Read the model definition and answer for the solid it produces. Units are mm, in the model's axes. Face numbers are marked on the shaded views. A direction names the side the tool comes from. Coordinates: 2 decimals unless noted, no trailing zeros. Write each loop counter-clockwise with the first axis right and the second up, starting at its lowest first coordinate (ties: lowest second). Pieces come first, ordered by that corner, then holes. Notation, with made-up numbers: (-11.75, -4) -> (-0.75, -4) arc R31 cw to (-0.75, 35) -> close; hole circle Ø2 at (14.25, 6.5). An arc over 180 degrees is marked (long way). One line per item, written item: value. Start each with the question number.
1. Consider line 1 along Y through (x, z) = (120, 7.5); line 2 along X through (y, z) = (460, 8); line 3 along Y through (x, z) = (304.5, -42). Determine where each line is inside the solid, lowest interval first.
2. Find section A-A, the plane x = 120. Write down the section's boundary in (y, z).
3. Find section D-D, the plane x = 200. Write down the section's boundary in (y, z), and give its area (3 significant figures).
4. Find section C-C, the plane y = 460. Write down the section's boundary in (x, z), and give its area (3 significant figures).
5. For the marked faces 1, 2 and 3, determine the directions among +Z, -Z, +X, -X, +Y, -Y from which every point of the face is accessible in a straight line to the end or side of a thin tool.
6. Find section B-B, the plane z = -41. Write down the section's boundary in (x, y).
7. Given P1, Ø15, axis at x = 282.5, z = -16, coming from the -Y side; P2, Ø15, axis at x = 296, z = -35.5, coming from the +Y side; P3, Ø8, axis at x = 312.5, y = 414.5, coming from the -Z side; P4, Ø10, axis at x = 148.5, z = -3, coming from the +Y side, each flat-ended and moving along its own axis, determine where each tip first touches the part or whether it passes through.
Autodesk Inventor part; units mm, degrees
ref_plane "YZ Plane" through (0, 0, 0) normal (1, 0, 0) x (0, 1, 0)
ref_plane "XZ Plane" through (0, 0, 0) normal (0, 1, 0) x (-1, 0, 0)
ref_plane "XY Plane" through (0, 0, 0) normal (0, 0, 1) x (1, 0, 0)
sketch "Sketch1" plane through (0, 0, 0) normal (0, 0, 1) x (1, 0, 0)
  line L0 (0, 0) -> (350, 0)
  line L1 (350, 0) -> (350, 520)
  line L2 (350, 520) -> (0, 520)
  line L3 (0, 520) -> (0, 0)
  dimension "d0" = 350
  dimension "d1" = 520
extrude "Extrusion1" add sketch "Sketch1" along normal blind 12
sketch "Sketch2" plane through (0, 0, 12) normal (0, 0, 1) x (1, 0, 0)
  line L0 (0, 120) -> (350, 120)
  line L1 (350, 120) -> (350, 370)
  line L2 (350, 0) -> (350, 520)
  line L3 (350, 370) -> (0, 370)
  line L4 (0, 520) -> (0, 0)
  line L5 (0, 370) -> (0, 520)
  line L6 (350, 520) -> (0, 520)
  line L7 (0, 520) -> (350, 520)
  line L8 (350, 520) -> (350, 370)
  circle A0 centre (120, 460) radius 6.5
  circle A1 centre (120, 250) radius 6.5
  dimension "d6" = 13
  dimension "d7" = 13
extrude "Extrusion2" cut sketch "Sketch2" against normal blind 12 contours A0 | A1
thread "Thread1"
thread "Thread2"
sketch "Sketch3" plane through (0, 0, 0) normal (0, 0, -1) x (-1, 0, 0)
  circle A0 centre (-200, 460) radius 6.5
  point P0 (0, 0)
  dimension "d14" = 13
extrude "Extrusion3" cut sketch "Sketch3" against normal blind 120
sketch "Sketch4" plane through (0, 0, 12) normal (0, 0, 1) x (1, 0, 0)
  point P0 (0, 0)
sketch "Sketch5" plane through (0, 0, 0) normal (0, 0, -1) x (-1, 0, 0)
  point P0 (0, 0)
sketch "Sketch6" plane through (0, 0, 0) normal (0, 0, -1) x (-1, 0, 0)
  line L0 (-330, 400) -> (-250, 400)
  line L1 (-250, 400) -> (-250, 360)
  line L2 (-250, 360) -> (-330, 360)
  line L3 (-330, 360) -> (-330, 400)
  line L4 (-330, 190) -> (-250, 190)
  line L5 (-250, 190) -> (-250, 150)
  line L6 (-250, 150) -> (-330, 150)
  line L7 (-330, 150) -> (-330, 190)
  point P0 (0, 0)
  dimension "d17" = 80
  dimension "d18" = 40
  dimension "d19" = 80
  dimension "d20" = 40
extrude "Extrusion4" add sketch "Sketch6" along normal blind 50
properties part number "back plate"
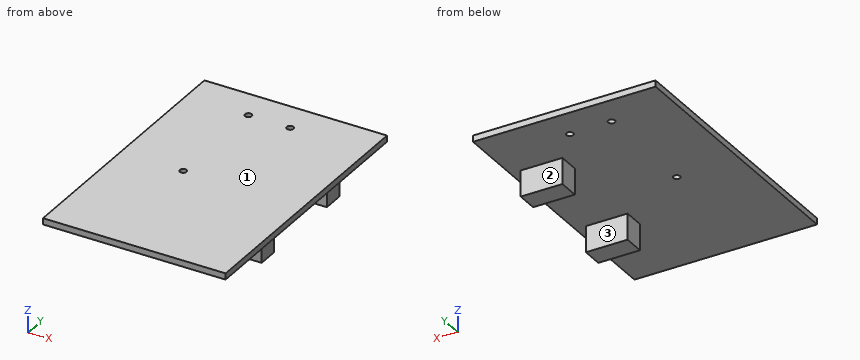
Answer block:
1. line 1: y = 0 to 243.5, 256.5 to 453.5, 466.5 to 520
1. line 2: x = 0 to 113.5, 126.5 to 193.5, 206.5 to 350
1. line 3: y = 150 to 190, 360 to 400
2. outline: (0, 0) -> (243.5, 0) -> (243.5, 12) -> (0, 12) -> close; (256.5, 0) -> (453.5, 0) -> (453.5, 12) -> (256.5, 12) -> close; (466.5, 0) -> (520, 0) -> (520, 12) -> (466.5, 12) -> close
3. outline: (0, 0) -> (453.5, 0) -> (453.5, 12) -> (0, 12) -> close; (466.5, 0) -> (520, 0) -> (520, 12) -> (466.5, 12) -> close
3. area: 6,080 mm2
4. outline: (0, 0) -> (113.5, 0) -> (113.5, 12) -> (0, 12) -> close; (126.5, 0) -> (193.5, 0) -> (193.5, 12) -> (126.5, 12) -> close; (206.5, 0) -> (350, 0) -> (350, 12) -> (206.5, 12) -> close
4. area: 3,890 mm2
5. face 1: +Z, +X, -X, +Y, -Y
5. face 2: -Z, +X, -X, +Y
5. face 3: -Z, +X, -X
6. outline: (250, 150) -> (330, 150) -> (330, 190) -> (250, 190) -> close; (250, 360) -> (330, 360) -> (330, 400) -> (250, 400) -> close
7. P1: stops at y = 150
7. P2: stops at y = 400
7. P3: stops at z = 0
7. P4: stops at y = 520
